from build123d import *

# Parameters (mm, degrees)
BOSS_EXTRUDE1_DEPTH = 1.5
FILLET5_R           = 2
CHAMFER1_SIZE       = 0.5


with BuildPart() as part:
    # Sketch1 → Boss-Extrude1 (new, symmetric)
    with BuildSketch(Plane(origin=(0, 0, 0), x_dir=(1, 0, 0), z_dir=(0, 1, 0))):
        Polygon((-14.297771125, -12.5), (14.297771125, -12.5), (22.216878365, -12.5), (7.783121635, 12.5), (-7.783121635, 12.5), (-22.216878365, -12.5), align=None)
    extrude(amount=BOSS_EXTRUDE1_DEPTH, both=True)

    # Fillet5
    fillet5_edges = [part.edges().sort_by_distance(p)[0] for p in [
        (-22.216878365, 0, 12.5),
        (-7.783121635, 0, -12.5),
        (7.783121635, 0, -12.5),
        (22.216878365, 0, 12.5),
    ]]
    fillet(fillet5_edges, radius=FILLET5_R)

    # Chamfer1
    chamfer1_edges = [part.edges().sort_by_distance(p)[0] for p in [
        (-14.422649731, -1.5, -1),
        (0, -1.5, 12.5),
        (0, -1.5, -12.5),
        (14.422649731, -1.5, -1),
        (-20.484827557, -1.5, 11.5),
        (20.484827557, -1.5, 11.5),
        (7.628421097, -1.5, -12.232050808),
        (-7.628421097, -1.5, -12.232050808),
    ]]
    chamfer(chamfer1_edges, length=CHAMFER1_SIZE)


solid = part.part
Check sheet for the modelled part. Datum: model origin and axes. Units: mm. Coordinates: 2 decimals unless noted, no trailing zeros. Loops run counter-clockwise (first coordinate to the right, second up) from the corner with the lowest first, then second, coordinate; pieces in that order, holes last. Notation, with made-up numbers: (62.25, 75) -> (102.25, 75) arc R24 cw to (102.25, 92) -> close; hole circle Ø9 at (-4, 17). An arc over 180 degrees is marked (long way). Answer in a Markdown table with one row per item.
1. Sectioned sample at B-B, the plane x = 10. Record the boundary of the cut face in (y, z), then the cut area to 3 significant figures.
Check values:
| item | result |
|---|---|
| outline | (-1.5, -7.66) -> (-1, -8.66) -> (1.5, -8.66) -> (1.5, 12.5) -> (-1, 12.5) -> (-1.5, 12) -> close |
| area | 63.1 mm2 |
2. Material ranges on line 1 along Z through (x, y) = (-8.5, 0.9); line 2 along X through (y, z) = (1.05, 2.25); line 3 along X through (y, z) = (1.4, 5.5), recorded low to high. Write a range as [from, to].
Check values:
| item | result |
|---|---|
| line 1 | z = [-11.26, 12.5] |
| line 2 | x = [-16.3, 16.3] |
| line 3 | x = [-18.18, 18.18] |
3. Sectioned sample at A-A, the plane y = -0.2. Record the boundary of the cut face in (x, z).
Check values:
| item | result |
|---|---|
| outline | (-20.48, 9.5) -> (-8.36, -11.5) arc R2 ccw to (-6.63, -12.5) -> (6.63, -12.5) arc R2 ccw to (8.36, -11.5) -> (20.48, 9.5) arc R2 ccw to (18.75, 12.5) -> (-18.75, 12.5) arc R2 ccw to start |
4. Sectioned sample at C-C, the plane z = -1. Record the boundary of the cut face in (x, y).
Check values:
| item | result |
|---|---|
| outline | (-14.42, -1) -> (-13.85, -1.5) -> (13.85, -1.5) -> (14.42, -1) -> (14.42, 1.5) -> (-14.42, 1.5) -> close |
